Here's how the part is built. I have some questions about the finished solid (model axes, mm). Face numbers are marked on the shaded views. A direction names the side the tool comes from. Coordinates: 2 decimals unless noted, no trailing zeros. Order: outer loops, then holes, each group sorted by start corner. A loop starts at its lowest first (then second) coordinate and runs counter-clockwise, first axis right, second up.
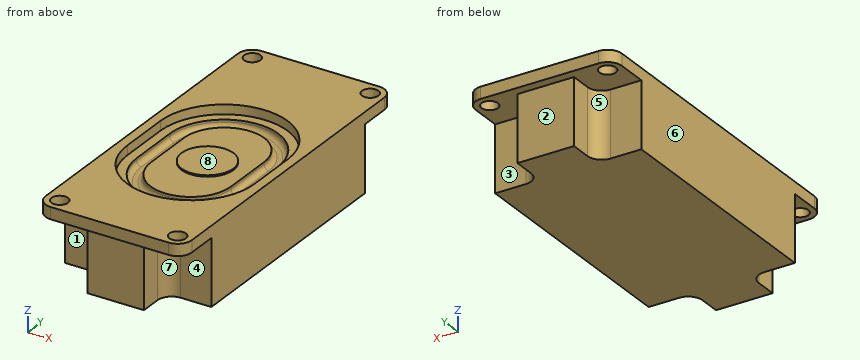
```python
from build123d import *

# Parameters (mm, degrees)
SKETCH_W        = 31
SKETCH_H        = 70
PAD_DEPTH       = 2.5
SKETCH001_R     = 1.75
POCKET_DEPTH    = 2.5
FILLET_R        = 3
PAD001_DEPTH    = 14
FILLET001_R     = 3
POCKET001_DEPTH = 2
POCKET002_DEPTH = 1.5
FILLET002_R     = 1
SKETCH005_R     = 5.5
PAD002_DEPTH    = 0.3


with BuildPart() as part:
    # Sketch → Pad (new body)
    with BuildSketch(Plane.XY):
        with Locations((0, 35)):
            Rectangle(SKETCH_W, SKETCH_H)
    extrude(amount=PAD_DEPTH)

    # Sketch001 (on Face6 of Pad) → Pocket (cut)
    with BuildSketch(Plane.XY.offset(2.5)):
        with Locations((-12.5, 67)):
            Circle(SKETCH001_R)
        with Locations((12.5, 67)):
            Circle(SKETCH001_R)
        with Locations((-12.5, 3)):
            Circle(SKETCH001_R)
        with Locations((12.5, 3)):
            Circle(SKETCH001_R)
    extrude(amount=-POCKET_DEPTH, mode=Mode.SUBTRACT)

    # Fillet
    fillet_edges = [part.edges().sort_by_distance(p)[0] for p in [
        (-15.5, 0, 1.25),
        (15.5, 0, 1.25),
        (-15.5, 70, 1.25),
        (15.5, 70, 1.25),
    ]]
    fillet(fillet_edges, radius=FILLET_R)

    # Sketch002 (on Face2 of Fillet) → Pad001 (join)
    with BuildSketch(Plane(origin=(0, 0, 0), x_dir=(1, 0, 0), z_dir=(0, 0, -1))):
        Polygon((-6, -2), (6, -2), (6, -9.5), (15.5, -9.5), (15.5, -60.5), (6, -60.5), (6, -68), (-6, -68), (-6, -60.5), (-15.5, -60.5), (-15.5, -9.5), (-6, -9.5), align=None)
    extrude(amount=PAD001_DEPTH)

    # Fillet001
    fillet001_edges = [part.edges().sort_by_distance(p)[0] for p in [
        (6, 9.5, -7),
        (-6, 9.5, -7),
        (-6, 60.5, -7),
        (6, 60.5, -7),
    ]]
    fillet(fillet001_edges, radius=FILLET001_R)

    # Sketch003 (on Face20 of Fillet001) → Pocket001 (cut)
    with BuildSketch(Plane.XY.offset(2.5)):
        with BuildLine():
            ThreePointArc((13.5, 38), (0, 51.5), (-13.5, 38))
            Line((-13.5, 38), (-13.5, 27))
            ThreePointArc((-13.5, 27), (0, 13.5), (13.5, 27))
            Line((13.5, 27), (13.5, 38))
        make_face()
    extrude(amount=-POCKET001_DEPTH, mode=Mode.SUBTRACT)

    # Sketch004 (on Face37 of Pocket001) → Pocket002 (cut)
    with BuildSketch(Plane.XY.offset(0.5)):
        with BuildLine():
            ThreePointArc((11.5, 38), (0, 49.5), (-11.5, 38))
            Line((-11.5, 38), (-11.5, 27))
            ThreePointArc((-11.5, 27), (0, 15.5), (11.5, 27))
            Line((11.5, 27), (11.5, 38))
        make_face()
        with BuildLine():
            ThreePointArc((8.5, 38), (0, 46.5), (-8.5, 38))
            Line((-8.5, 38), (-8.5, 27))
            ThreePointArc((-8.5, 27), (0, 18.5), (8.5, 27))
            Line((8.5, 27), (8.5, 38))
        make_face(mode=Mode.SUBTRACT)
    extrude(amount=-POCKET002_DEPTH, mode=Mode.SUBTRACT)

    # Fillet002
    fillet002_edges = [part.edges().sort_by_distance(p)[0] for p in [
        (0, 49.5, -1),
        (0, 15.5, -1),
        (-11.5, 32.5, -1),
        (0, 46.5, -1),
        (8.5, 32.5, -1),
        (0, 18.5, -1),
        (-8.5, 32.5, -1),
        (11.5, 32.5, -1),
    ]]
    fillet(fillet002_edges, radius=FILLET002_R)

    # Sketch005 (on Face36 of Fillet002) → Pad002 (join)
    with BuildSketch(Plane.XY.offset(0.5)):
        with Locations((0, 32.5)):
            Circle(SKETCH005_R)
    extrude(amount=PAD002_DEPTH)


solid = part.part
```
Q1. I need wall thicknesses on L1, parallel to X at y = 67, z = 0.75; L2, parallel to Y at x = 5, z = -0.75; L3, parallel to Y at x = 2.5, z = -0.75. Which ranges of each line are inside material? Lowest first, please.
Q2. For the marked faces 1, 2, 3, 4 and 5, which set-ups out of +Z, -Z, +X, -X, +Y, -Y let a thin tool reach every point of the face, with its end or its side?
Q3. We'd pull the mould along X, two halves only. Please class the marked faces 6, 7 and 8: pulls with the +X half, pulls with the -X half, needs draft (parallel to the pull), parting line crosses it, or undercut.
Q4. If we section it at D-D on y = 64.5: Write out the boundary of the cut face in (x, z).
Q5. Will these pins go through, and if not, where does the flat tip stop? pin 1 (5 mm diameter, centred on y = 5.5, z = -8.5, fed in from -X); pin 2 (8 mm diameter, centred on x = -5.5, z = -9.5, fed in from +Y); pin 3 (6 mm diameter, centred on x = -2.5, z = -10, fed in from -Y); pin 4 (3 mm diameter, centred on x = 12.5, y = 67, fed in from +Z).
Q6. If we section it at C-C on x = 0: Write out the boundary of the cut face in (y, z), then the cut area to 3 significant figures.
Q7. If we section it at B-B on y = 32.5: Write out the boundary of the cut face in (x, z).
Q8. If we section it at A-A on z = -5.75: Write out the boundary of the cut face in (x, y).
Reply:
1. L1: x = -15.5 to -14.25, -10.75 to 10.75, 14.25 to 15.5
1. L2: y = 2 to 17.02, 19.71 to 45.29, 47.98 to 68
1. L3: y = 2 to 16.12, 18.52 to 46.48, 48.88 to 68
2. face 1: -Z, -X, -Y
2. face 2: -Z, +X, -X, +Y
2. face 3: -Z, +X, +Y
2. face 4: -Z, +X, -Y
2. face 5: -Z, -X, +Y
3. face 6: pulls with the -X half
3. face 7: pulls with the +X half
3. face 8: undercut
4. outline: (-15.5, 0) - (-6, 0) - (-6, -14) - (6, -14) - (6, 0) - (15.5, 0) - (15.5, 2.5) - (-15.5, 2.5) - close
5. pin 1: stops at x = -6.4
5. pin 2: stops at y = 68
5. pin 3: stops at y = 2
5. pin 4: passes through
6. outline: (0, 0) - (2, 0) - (2, -14) - (68, -14) - (68, 0) - (70, 0) - (70, 2.5) - (51.5, 2.5) - (51.5, 0.5) - (49.5, 0.5) - (49.5, 0) arc R1 cw to (48.5, -1) - (47.5, -1) arc R1 cw to (46.5, 0) - (46.5, 0.5) - (38, 0.5) - (38, 0.8) - (27, 0.8) - (27, 0.5) - (18.5, 0.5) - (18.5, 0) arc R1 cw to (17.5, -1) - (16.5, -1) arc R1 cw to (15.5, 0) - (15.5, 0.5) - (13.5, 0.5) - (13.5, 2.5) - (0, 2.5) - close
6. area: 1,020 mm2
7. outline: (-15.5, -14) - (15.5, -14) - (15.5, 2.5) - (13.5, 2.5) - (13.5, 0.5) - (11.5, 0.5) - (11.5, 0) arc R1 cw to (10.5, -1) - (9.5, -1) arc R1 cw to (8.5, 0) - (8.5, 0.5) - (5.5, 0.5) - (5.5, 0.8) - (-5.5, 0.8) - (-5.5, 0.5) - (-8.5, 0.5) - (-8.5, 0) arc R1 cw to (-9.5, -1) - (-10.5, -1) arc R1 cw to (-11.5, 0) - (-11.5, 0.5) - (-13.5, 0.5) - (-13.5, 2.5) - (-15.5, 2.5) - close
8. outline: (-15.5, 9.5) - (-9, 9.5) arc R3 cw to (-6, 6.5) - (-6, 2) - (6, 2) - (6, 6.5) arc R3 cw to (9, 9.5) - (15.5, 9.5) - (15.5, 60.5) - (9, 60.5) arc R3 cw to (6, 63.5) - (6, 68) - (-6, 68) - (-6, 63.5) arc R3 cw to (-9, 60.5) - (-15.5, 60.5) - close
